Design review of the part built by this model. Coordinates are the model's own, in mm. A direction names the side the tool comes from. Coordinates: 2 decimals unless noted, no trailing zeros. Write each loop counter-clockwise with the first axis right and the second up, starting at its lowest first coordinate (ties: lowest second). Pieces come first, ordered by that corner, then holes. Notation, with made-up numbers: (75.5, 68.5) -> (107.5, 68.5) arc R25 ccw to (107.5, 104.5) -> close; hole circle Ø10 at (-27.5, 19). An arc over 180 degrees is marked (long way). One line per question, with ' | ' between items. Start each with the question number.
Q1. Add section B-B on z = 2.5. State the section outline as (x, y) points.
Q2. Add section D-D on z = 3.3. State the section outline as (x, y) points, and give its area (3 significant figures).
Q3. For P1, Ø1.6, axis at y = 1.5, z = 3.5, coming from the +X side; P2, Ø1, axis at x = -7, z = 1.5, coming from the +Y side, all flat-tipped, find the tip position at first contact; note any pin that passes through.
Q4. Add section C-C on y = 2.25. State the section outline as (x, z) points, and give its area (3 significant figures).
Q5. For faces 1 (the flat face through (-9, 0, 2)), 2 (the flat face through (-9, 0.5, 2)), 3 (the flat face through (0, 3.5, 2)), 4 (the flat face through (5, 2, 2)), 5 (the flat face through (9, 0.5, 2)), list the 3-axis set-ups (+Z, -Z, +X, -X, +Y, -Y) from which the entire face can be reached by the end or side of a thin tool; tool diameter is ignored.
Q6. Wall thickness on probe 1 along Z at (x, y) = (-7.5, 0.2); probe 2 along X at (y, z) = (1.2, 2.95); probe 3 along Y at (x, z) = (0.5, 3): over which ranges is each line inside the solid? List them lowest first.
Q7. Add section A-A on x = 7.5. State the section outline as (y, z) points, and give its area (3 significant figures).
Q8. Draft analysis for pull direction Z (two halves, no side actions). For faces 6 (the cylindrical face through (-6.5, 0.3, 2.5)), 7 (the flat face through (0, 3.2, 0)), 8 (the flat face through (0, 3.2, 5)), 9 (the flat face through (9, 0, 2)), state which applies: pulls with the +Z half, pulls with the -Z half, needs draft (parallel to the pull), parting line crosses it, or undercut.
from build123d import *

# Parameters (mm, degrees)
BASE_FLANGE1_DEPTH = 5
SKETCH7_R          = 1
CUT_EXTRUDE1_DEPTH = 10


# Sheet-metal steps are written as plain solids
with BuildPart() as part:
    # Sketch2 → Base-Flange1 (new body)
    with BuildSketch(Plane.XY):
        with BuildLine():
            Line((-9.5, 0), (-6, 0))
            ThreePointArc((-6, 0), (-5.292893219, 0.292893219), (-5, 1))
            Line((-5, 1), (-5, 2.5))
            ThreePointArc((-5, 2.5), (-4.853553391, 2.853553391), (-4.5, 3))
            Line((-4.5, 3), (4.5, 3))
            ThreePointArc((4.5, 3), (4.853553391, 2.853553391), (5, 2.5))
            Line((5, 2.5), (5, 1))
            ThreePointArc((5, 1), (5.292893219, 0.292893219), (6, 0))
            Line((6, 0), (9.5, 0))
            Line((9.5, 0), (9.5, 0.5))
            Line((9.5, 0.5), (6, 0.5))
            ThreePointArc((6, 0.5), (5.646446609, 0.646446609), (5.5, 1))
            Line((5.5, 1), (5.5, 2.5))
            ThreePointArc((5.5, 2.5), (5.207106781, 3.207106781), (4.5, 3.5))
            Line((4.5, 3.5), (-4.5, 3.5))
            ThreePointArc((-4.5, 3.5), (-5.207106781, 3.207106781), (-5.5, 2.5))
            Line((-5.5, 2.5), (-5.5, 1))
            ThreePointArc((-5.5, 1), (-5.646446609, 0.646446609), (-6, 0.5))
            Line((-6, 0.5), (-9.5, 0.5))
            Line((-9.5, 0.5), (-9.5, 0))
        make_face()
    extrude(amount=BASE_FLANGE1_DEPTH)

    # Sketch7 → Cut-Extrude1 (cut)
    with BuildSketch(Plane(origin=(0, 0.5, 0), x_dir=(1, 0, 0), z_dir=(0, 1, 0))):
        with Locations(Location((-7.5, -2.5, 0), (0, 0, 180))):
            Circle(SKETCH7_R)
        with Locations((7.5, -2.5)):
            Circle(SKETCH7_R)
    extrude(amount=-CUT_EXTRUDE1_DEPTH, mode=Mode.SUBTRACT)


solid = part.part
Output values:
1) outline: (-9.5, 0) -> (-8.5, 0) -> (-8.5, 0.5) -> (-9.5, 0.5) -> close; (-6.5, 0) -> (-6, 0) arc R1 ccw to (-5, 1) -> (-5, 2.5) arc R0.5 cw to (-4.5, 3) -> (4.5, 3) arc R0.5 cw to (5, 2.5) -> (5, 1) arc R1 ccw to (6, 0) -> (6.5, 0) -> (6.5, 0.5) -> (6, 0.5) arc R0.5 cw to (5.5, 1) -> (5.5, 2.5) arc R1 ccw to (4.5, 3.5) -> (-4.5, 3.5) arc R1 ccw to (-5.5, 2.5) -> (-5.5, 1) arc R0.5 cw to (-6, 0.5) -> (-6.5, 0.5) -> close; (8.5, 0) -> (9.5, 0) -> (9.5, 0.5) -> (8.5, 0.5) -> close
2) outline: (-9.5, 0) -> (-8.1, 0) -> (-8.1, 0.5) -> (-9.5, 0.5) -> close; (-6.9, 0) -> (-6, 0) arc R1 ccw to (-5, 1) -> (-5, 2.5) arc R0.5 cw to (-4.5, 3) -> (4.5, 3) arc R0.5 cw to (5, 2.5) -> (5, 1) arc R1 ccw to (6, 0) -> (6.9, 0) -> (6.9, 0.5) -> (6, 0.5) arc R0.5 cw to (5.5, 1) -> (5.5, 2.5) arc R1 ccw to (4.5, 3.5) -> (-4.5, 3.5) arc R1 ccw to (-5.5, 2.5) -> (-5.5, 1) arc R0.5 cw to (-6, 0.5) -> (-6.9, 0.5) -> close; (8.1, 0) -> (9.5, 0) -> (9.5, 0.5) -> (8.1, 0.5) -> close | area: 10.7 mm2
3) P1: stops at x = 5.6 | P2: stops at y = 0.5
4) outline: (-5.5, 0) -> (-5, 0) -> (-5, 5) -> (-5.5, 5) -> close; (5, 0) -> (5.5, 0) -> (5.5, 5) -> (5, 5) -> close | area: 5.00 mm2
5) face 1: +Z, -Z, +X, -X, -Y | face 2: +Z, -Z, -X, +Y | face 3: +Z, -Z, +X, -X, +Y | face 4: +Z, -Z, -Y | face 5: +Z, -Z, +X, +Y
6) probe 1: z = 0 to 1.5, 3.5 to 5 | probe 2: x = -5.5 to -5, 5 to 5.5 | probe 3: y = 3 to 3.5
7) outline: (0, 0) -> (0.5, 0) -> (0.5, 1.5) -> (0, 1.5) -> close; (0, 3.5) -> (0.5, 3.5) -> (0.5, 5) -> (0, 5) -> close | area: 1.50 mm2
8) face 6: undercut | face 7: pulls with the -Z half | face 8: pulls with the +Z half | face 9: needs draft
